For this review, take the finished solid that the model builds, in its own axes (mm). A direction names the side the tool comes from. Give positions to 0.01 mm unless a question says otherwise; leave off trailing zeros. Write each loop counter-clockwise with the first axis right and the second up, starting at its lowest first coordinate (ties: lowest second). Pieces come first, ordered by that corner, then holes.
Q1. Machinability: for faces 5 (the flat face through (-2, 7, 2)), 6 (the conical face through (-1.206, -5.433, 17.212)), 7 (the cylindrical face through (-7.85, -4.4, 2.99)), which of the approach directions +Z, -Z, +X, -X, +Y, -Y give a long, thin tool a straight path to every point of the face, cutting with its end or side? Answer none if there is none.
Q2. We need section A-A (x = 0). Write out the cut boundary in (y, z), then the cut area to 3 significant figures.
Q3. Insertion check: P1, Ø5, axis at y = -5, z = 17.5, coming from the -X side; P2, Ø6, axis at x = -6, z = 5, coming from the -Y side; P3, Ø5, axis at y = 3.5, z = 6, coming from the -X side. Each pin has a flat end and moves straight along its axis. Give the tip position at first contact, or say it passes through.
Q4. We need section B-B (z = 3). Write out the cut boundary in (x, y) (3 decimals).
Q5. For line 1 (Z direction, x = 1.75, y = -1); line 2 (X direction, y = -1, z = 31); line 3 (Y direction, x = -0.5, z = 32), list the stretches that pass through material, from the lowest coordinate up.
Q6. We need section D-D (z = 19). Write out the cut boundary in (x, y), then the cut area to 3 significant figures.
Q7. Mouldability with a two-part tool opening along Y and no side actions: class faces 1 (the cylindrical face through (6.511, 3.723, 4.967)), 2 (the cylindrical face through (0, 9, 3)), 3 (the cylindrical face through (0, -7.5, 5)), 4 (the flat face through (0, 0, 29)) as released by +Y, released by -Y, zero draft, split by the parting line, or undercut.
Q8. We need section C-C (z = 30.5). Write out the cut boundary in (x, y).
```python
from build123d import *

# Parameters (mm, degrees)
F0_R      = 7
F1_DEPTH  = 2
F2_R      = 9
F2_R_2    = 7
F3_DEPTH  = 2
F3_FACE_R = 9
F5_R      = 2.5
F10_DEPTH = 32.001


with BuildPart() as f1:
    # F0 (on Top) → F1 (new body)
    with BuildSketch(Plane.XY):
        Circle(F0_R)
    extrude(amount=F1_DEPTH)

    # F2 (on face) → F3 (join)
    with BuildSketch(Plane.XY.offset(2)):
        Circle(F2_R)
        Circle(F2_R_2, mode=Mode.SUBTRACT)
        Circle(F2_R_2)
    extrude(amount=F3_DEPTH)

    # F3_face (on face) → F6 section 0
    with BuildSketch(Plane.XY.offset(4)):
        Circle(F3_FACE_R)
    # F5 (on offset) → F6 section 1
    with BuildSketch(Plane.XY.offset(29)):
        Circle(F5_R)
    loft()

    # F7 (on face) → F8 (revolve)
    with BuildSketch(Plane.XY.offset(29)):
        with BuildLine():
            ThreePointArc((0, -5), (3.5355339059, -3.5355339059), (5, 0))
            ThreePointArc((5, 0), (3.5355339059, 3.5355339059), (0, 5))
            Line((0, 5), (0, 2.5))
            ThreePointArc((0, 2.5), (1.767766953, 1.767766953), (2.5, 0))
            ThreePointArc((2.5, 0), (1.767766953, -1.767766953), (0, -2.5))
            Line((0, -2.5), (0, -5))
        make_face()
    revolve(axis=Axis((0, 0, 29), (0, -1, 0)))

    # F9 (on face) → F10 (cut, through all)
    with BuildSketch(Plane(origin=(0, 0, 2), x_dir=(1, 0, 0), z_dir=(0, 0, -1))):
        with BuildLine():
            ThreePointArc((1.4947825929, 8.875), (0, 9), (-1.4947825929, 8.875))
            ThreePointArc((-1.4947825929, 8.875), (0, 7.5), (1.4947825929, 8.875))
        make_face()
        with BuildLine():
            ThreePointArc((1.4947825929, 8.875), (1.4986950806, 8.937445581), (1.5, 9))
            ThreePointArc((1.5, 9), (-0.062554419, 10.4986950806), (-1.4947825929, 8.875))
            ThreePointArc((-1.4947825929, 8.875), (0, 9), (1.4947825929, 8.875))
        make_face()
        with BuildLine():
            ThreePointArc((6.9385841621, -5.7320196986), (7.7942286341, -4.5), (8.433366755, -3.1429803014))
            ThreePointArc((8.433366755, -3.1429803014), (6.4951905284, -3.75), (6.9385841621, -5.7320196986))
        make_face()
        with BuildLine():
            ThreePointArc((9.2942286341, -4.5), (9.0608594369, -3.6964787437), (8.433366755, -3.1429803014))
            ThreePointArc((8.433366755, -3.1429803014), (7.7942286341, -4.5), (6.9385841621, -5.7320196986))
            ThreePointArc((6.9385841621, -5.7320196986), (8.4894024584, -5.8291852218), (9.2942286341, -4.5))
        make_face()
        with BuildLine():
            ThreePointArc((-6.2942286341, -4.5), (-6.9907073778, -3.2333691972), (-8.433366755, -3.1429803014))
            ThreePointArc((-8.433366755, -3.1429803014), (-7.7942286341, -4.5), (-6.9385841621, -5.7320196986))
            ThreePointArc((-6.9385841621, -5.7320196986), (-6.4650434122, -5.1951738244), (-6.2942286341, -4.5))
        make_face()
        with BuildLine():
            ThreePointArc((-6.9385841621, -5.7320196986), (-7.7942286341, -4.5), (-8.433366755, -3.1429803014))
            ThreePointArc((-8.433366755, -3.1429803014), (-9.0932667397, -5.25), (-6.9385841621, -5.7320196986))
        make_face()
    extrude(amount=-F10_DEPTH, mode=Mode.SUBTRACT)


solid = f1.part
```
Computed:
1. face 5: -Z
1. face 6: none
1. face 7: +Z, -Z, -X
2. outline: (-7.5, 2) - (-7, 2) - (-7, 0) - (7, 0) - (7, 2) - (9, 2) - (9, 4) - (3.44, 25.37) arc R5 ccw (long way) to (-3.44, 25.37) - (-7.5, 9.77) - close; hole (-2.5, 29) - (2.5, 29) arc R2.5 ccw to start
2. area: 385 mm2
3. P1: stops at x = -5.08
3. P2: stops at y = -8.42
3. P3: stops at x = -8.78
4. outline: (-8.433, 3.143) arc R9 ccw to (-1.495, -8.875) arc R1.5 cw to (1.495, -8.875) arc R9 ccw to (8.433, 3.143) arc R1.5 cw to (6.939, 5.732) arc R9 ccw to (-6.939, 5.732) arc R1.5 cw to start
5. line 1: z = 0 to 29, 30.48 to 33.58
5. line 2: x = -4.47 to -1.12, 1.12 to 4.47
5. line 3: y = -3.97 to 3.97
6. outline: circle Ø10.2 at (0, 0)
6. area: 81.7 mm2
7. face 1: undercut
7. face 2: released by +Y
7. face 3: released by -Y
7. face 4: undercut
8. outline: circle Ø9.54 at (0, 0); hole circle Ø4 at (0, 0)
